For this review, take the finished solid that the model builds, in its own axes (mm). Face numbers are marked on the shaded views. A direction names the side the tool comes from. Give positions to 0.01 mm unless a question says otherwise; leave off trailing zeros. Loops run counter-clockwise (first coordinate to the right, second up) from the corner with the lowest first, then second, coordinate; pieces in that order, holes last. Notation, with made-up numbers: (32, 69) -> (86, 69) arc R4 cw to (86, 74) -> close; hole circle Ø10 at (83, 68.25). An arc over 180 degrees is marked (long way). Answer as CSV lines item,"result". Start each with the question number.
Item 1: Add section A-A on z = 12. State how many separate pieces and enclosed holes the cut face has, plus the area to 3 significant figures.
Item 2: Machinability: for the marked faces 1, 2 and 3, which of the approach directions +Z, -Z, +X, -X, +Y, -Y give a long, thin tool a straight path to every point of the face, cutting with its end or side? Answer none if there is none.
Item 3: Add section B-B on y = -11.5. State the section outline as (x, z) points, plus the area to 3 significant figures.
Item 4: Clearance check with flat-ended pins moving along their axes: P1, Ø4, axis at x = 3.5, z = 10.5, coming from the -Y side; P2, Ø1.6, axis at y = 16, z = 7.5, coming from the +X side; P3, Ø0.6, axis at y = -19, z = 11.5, coming from the -X side. State where each tip first meets the part, or that it passes through.
Item 5: For L1, parallel to X at y = -19, z = 3.25; L2, parallel to Z at x = 15, y = 17, list the stretches that pass through material, from the lowest coordinate up. Write a range as from..to.
Item 6: Add section C-C on y = -17.5. State the section outline as (x, z) points, plus the area to 3 significant figures.
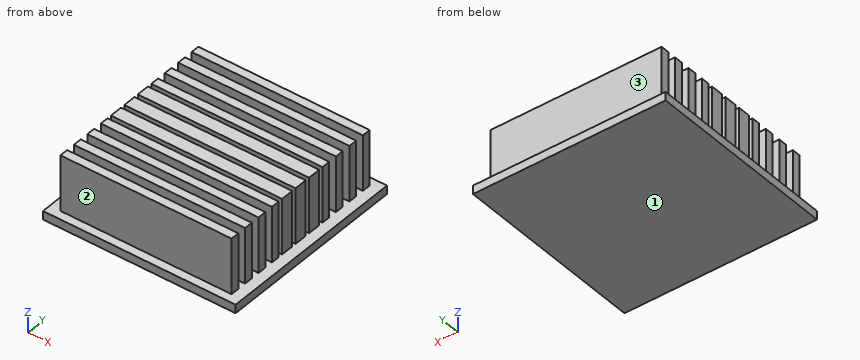
```python
from build123d import *

# Parameters (mm, degrees)
F0_W     = 45
F0_H     = 45
F1_DEPTH = 15
F2_W     = 45
F2_H     = 45
F2_W_2   = 40
F2_H_2   = 2
F3_DEPTH = 13


with BuildPart() as f1:
    # F0 (on Top) → F1 (new body)
    with BuildSketch(Plane.XY):
        Rectangle(F0_W, F0_H)
    extrude(amount=F1_DEPTH)

    # F2 (on face) → F3 (cut)
    with BuildSketch(Plane.XY.offset(15)):
        Rectangle(F2_W, F2_H)
        with Locations((0, -19.5)):
            Rectangle(F2_W_2, F2_H_2, mode=Mode.SUBTRACT)
        with Locations((0, -15.5)):
            Rectangle(F2_W_2, F2_H_2, mode=Mode.SUBTRACT)
        with Locations((0, -11.5)):
            Rectangle(F2_W_2, F2_H_2, mode=Mode.SUBTRACT)
        with Locations((0, -7.5)):
            Rectangle(F2_W_2, F2_H_2, mode=Mode.SUBTRACT)
        Polygon((-20, -4.5), (-20, -3.5), (-20, -2.5), (20, -2.5), (20, -3.5), (20, -4.5), (20, -5.5), (-20, -5.5), align=None, mode=Mode.SUBTRACT)
        Polygon((-20, -0.5), (-20, 0.5), (-20, 1.5), (20, 1.5), (20, 0.5), (20, -0.5), (20, -1.5), (-20, -1.5), align=None, mode=Mode.SUBTRACT)
        Polygon((-20, 3.5), (-20, 4.5), (-20, 5.5), (20, 5.5), (20, 4.5), (20, 3.5), (20, 2.5), (-20, 2.5), align=None, mode=Mode.SUBTRACT)
        with Locations((0, 7.5)):
            Rectangle(F2_W_2, F2_H_2, mode=Mode.SUBTRACT)
        with Locations((0, 11.5)):
            Rectangle(F2_W_2, F2_H_2, mode=Mode.SUBTRACT)
        with Locations((0, 15.5)):
            Rectangle(F2_W_2, F2_H_2, mode=Mode.SUBTRACT)
        with Locations((0, 19.5)):
            Rectangle(F2_W_2, F2_H_2, mode=Mode.SUBTRACT)
    extrude(amount=-F3_DEPTH, mode=Mode.SUBTRACT)


solid = f1.part
```
Computed values:
1,separate pieces,"11"
1,enclosed holes,"0"
1,area,"1,000 mm²"
2,face 1,"-Z, +X, -X, +Y, -Y"
2,face 2,"+Z, +X, -X, -Y"
2,face 3,"+Z, +X, -X, +Y"
3,outline,"(-22.5, 0) -> (22.5, 0) -> (22.5, 2) -> (20, 2) -> (20, 15) -> (-20, 15) -> (-20, 2) -> (-22.5, 2) -> close"
3,area,"610 mm²"
4,P1,"y = -20.5"
4,P2,"x = 20"
4,P3,"x = -20"
5,L1,"-20..20"
5,L2,"0..2"
6,outline,"(-22.5, 0) -> (22.5, 0) -> (22.5, 2) -> (-22.5, 2) -> close"
6,area,"90.0 mm²"
